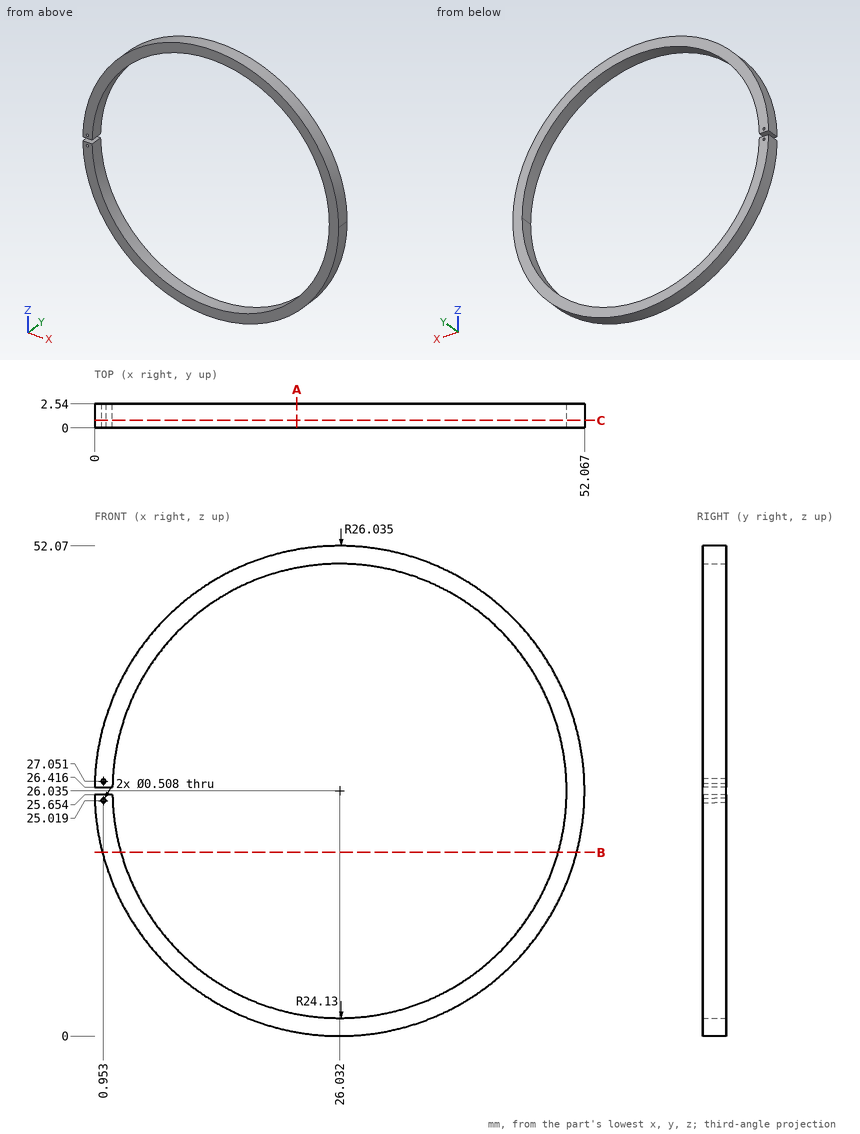
Job drawing, mm, ordinate dimensions from the low corner. One solid piece. Round coordinates to 2 decimals unless told otherwise and drop trailing zeros. Write each loop counter-clockwise with the first axis right and the second up, starting at its lowest first coordinate (ties: lowest second). Pieces come first, ordered by that corner, then holes. Notation, with made-up numbers: (70.5, 17) -> (87.5, 17) arc R17 cw to (87.5, 49) -> close; hole circle Ø7 at (60, 21.25). An arc over 180 degrees is marked (long way). Answer as a JSON object with one key per item and string values.
(1) Band-saw the part on C-C, the plane y = 0.8. List the corners of the cut face in (x, z) (1 decimal).
Reported:
{"outline": "(0, 25.7) arc R26 ccw (long way) to (0, 26.4) -> (1.9, 26.4) arc R24.1 cw (long way) to (1.9, 25.7) -> close; hole circle Ø0.5 at (1, 25); hole circle Ø0.5 at (1, 27.1)"}
(2) Probe probe 1 along X at (y, z) = (0.9, 26.5); probe 2 along Z at (x, y) = (26.5, 0.8) (1 decimal); probe 3 along X at (y, z) = (1.55, 25) (1 decimal). List the from-to ranges inside material, lowest first. Write a range as [from, to].
Reported:
{"probe 1": "x = [0, 1.91], [50.16, 52.06]", "probe 2": "z = [0, 1.9], [50.2, 52.1]", "probe 3": "x = [0, 0.7], [1.2, 1.9], [50.1, 52]"}
(3) Band-saw the part on A-A, the plane x = 21.5. List the corners of the cut face in (y, z) (1 decimal).
Reported:
{"outline": "(0, 0.4) -> (2.5, 0.4) -> (2.5, 2.3) -> (0, 2.3) -> close; (0, 49.7) -> (2.5, 49.7) -> (2.5, 51.7) -> (0, 51.7) -> close"}
(4) Pin check, flat tips, straight feed: P1, Ø6, axis at x = 14.5, z = 6, coming from the +Y side; P2, Ø1.5, axis at x = 29.5, y = 0.5, coming from the -Z side. Stop position of each tip, or through.
Reported:
{"P1": "stops at y = 2.54", "P2": "stops at z = 0.14"}
(5) Band-saw the part on B-B, the plane z = 19.5. List the corners of the cut face in (x, y).
Reported:
{"outline": "(0.83, 0) -> (2.8, 0) -> (2.8, 2.54) -> (0.83, 2.54) -> close; (49.26, 0) -> (51.23, 0) -> (51.23, 2.54) -> (49.26, 2.54) -> close"}
